from build123d import *

# Parameters (mm, degrees)
EXTRUDE1_START     = -6
SKETCH1_R          = 3
EXTRUDE1_DEPTH     = 14
EXTRUDE2_START     = -8
SKETCH6_R          = 5
EXTRUDE2_DEPTH     = 2
CUT_EXTRUDE1_DEPTH = 1.5
SKETCH8_R          = 2.309401077
CUT_EXTRUDE2_DEPTH = 1.5
CUT_EXTRUDE2_TAPER = 45
CHAMFER1_SIZE      = 0.25
CHAMFER2_SIZE      = 0.75


with BuildPart() as part:
    # Sketch1 → Extrude1 (new body)
    with BuildSketch(Plane.XY.offset(EXTRUDE1_START)):
        Circle(SKETCH1_R)
    extrude(amount=EXTRUDE1_DEPTH)

    # Sketch6 → Extrude2 (add)
    with BuildSketch(Plane.XY.offset(EXTRUDE2_START)):
        Circle(SKETCH6_R)
    extrude(amount=EXTRUDE2_DEPTH)

    # Sketch7 → Cut-Extrude1 (cut)
    with BuildSketch(Plane.XY.offset(-8)):
        Polygon((0, 2.309401077), (-2, 1.154700538), (-2, -1.154700538), (0, -2.309401077), (2, -1.154700538), (2, 1.154700538), align=None)
    extrude(amount=CUT_EXTRUDE1_DEPTH, mode=Mode.SUBTRACT)

    # Sketch8 → Cut-Extrude2 (cut)
    with BuildSketch(Plane.XY.offset(-8)):
        Circle(SKETCH8_R)
    extrude(amount=CUT_EXTRUDE2_DEPTH, taper=CUT_EXTRUDE2_TAPER, mode=Mode.SUBTRACT)

    # Chamfer1
    chamfer1_edges = [part.edges().sort_by_distance(p)[0] for p in [
        (-5, 0, -6),
        (-5, 0, -8),
    ]]
    chamfer(chamfer1_edges, length=CHAMFER1_SIZE)

    # Chamfer2
    chamfer2_edges = [part.edges().sort_by_distance(p)[0] for p in [
        (-3, 0, 8),
    ]]
    chamfer(chamfer2_edges, length=CHAMFER2_SIZE)


solid = part.part
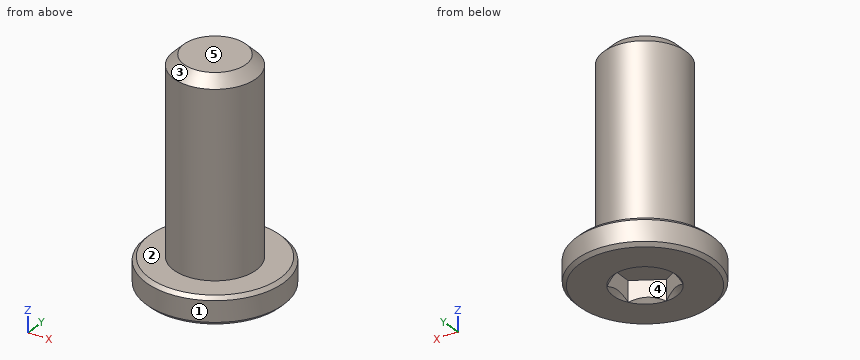
Can you work these out from the model? Positions are in its coordinate system, mm. Face numbers are marked on the shaded views. A direction names the side the tool comes from. Give positions to 0.01 mm unless a question says otherwise; leave off trailing zeros. Order: outer loops, then holes, each group sorted by start corner. A loop starts at its lowest first (then second) coordinate and runs counter-clockwise, first axis right, second up. Notation, with made-up numbers: M -38,-22.75 L 16,-22.75 A35 cw 16,12.25 Z; hole C 10,19 d4. An arc over 180 degrees is marked long. Use one line per item in the form item = value.
Item 1: If we section it at A-A, the plane y = 0: Write out the boundary of the cut face in (x, z), and give its area (3 significant figures).
Values follow:
outline = M -5,-7.75 L -4.75,-8 L -2.31,-8 L -2,-7.69 L -2,-6.5 L 2,-6.5 L 2,-7.69 L 2.31,-8 L 4.75,-8 L 5,-7.75 L 5,-6.25 L 4.75,-6 L 3,-6 L 3,7.25 L 2.25,8 L -2.25,8 L -3,7.25 L -3,-6 L -4.75,-6 L -5,-6.25 Z
area = 97.2 mm^2
Item 2: If we section it at B-B, the plane z = 1.5: Write out the boundary of the cut face in (x, y).
Values follow:
outline = C 0,0 d6
Item 3: Will these pins go through, and if not, where does the flat tip stop? pin 1 Ø6 at (x, z) = (-0.5, 2.5) entering from -Y; pin 2 Ø3 at (y, z) = (3, -2.5) entering from +X; pin 3 Ø4.5 at (x, y) = (0.5, -1) entering from -Z; pin 4 Ø1.5 at (x, z) = (-1.5, -2) entering from -Y.
Values follow:
pin_1 = -3
pin_2 = 2.6
pin_3 = -8
pin_4 = -2.9
Item 4: If I drill on line 1 along Z through (x, y) = (0, 2); line 2 along Z through (x, y) = (2.5, -2.75); line 3 along Y through (x, z) = (1, -7), over which ranges is the centre line in solid material (lowest first)? Write a range as [from, to].
Values follow:
line_1 = [-6.5, 8]
line_2 = [-8, -6]
line_3 = [-4.9, -1.73], [1.73, 4.9]
Item 5: For the marked faces 1 and 2, which set-ups out of +Z, -Z, +X, -X, +Y, -Y let a thin tool reach every point of the face, with its end or its side?
Values follow:
face_1 = +Z, -Z
face_2 = +Z
Item 6: Thinking about a two-plate mould opening in X: for the marked faces 3, 4 and 5, which applies, pulls with the +X half, pulls with the -X half, needs draft (parallel to the pull), parting line crosses it, or undercut?
Values follow:
face_3 = parting line crosses it
face_4 = undercut
face_5 = needs draft
